Build history of the part. All positions in model axes, mm. Give positions to 0.01 mm unless a question says otherwise; leave off trailing zeros. Write each loop counter-clockwise with the first axis right and the second up, starting at its lowest first coordinate (ties: lowest second). Pieces come first, ordered by that corner, then holes.
from build123d import *

# Parameters (mm, degrees)
BOSS_EXTRUDE1_DEPTH = 25.4
CUT_EXTRUDE2_DEPTH  = 23.957211
SKETCH4_R           = 2.159
BOSS_EXTRUDE2_DEPTH = 7.62


with BuildPart() as part:
    # Sketch1 → Boss-Extrude1 (new body)
    with BuildSketch(Plane.XY):
        with BuildLine():
            ThreePointArc((-160.997616832, 14.9225), (-115.11071, 26.01979846), (-79.36572698, 56.858969015))
            ThreePointArc((-79.36572698, 56.858969015), (-44.613051666, 86.842020921), (0, 97.63125))
            Line((0, 97.63125), (0, 84.93125))
            ThreePointArc((0, 84.93125), (-58.347374184, 61.716295679), (-84.797616832, 4.7625))
            Line((-84.797616832, 4.7625), (-160.997616832, 4.7625))
            Line((-160.997616832, 4.7625), (-160.997616832, 14.9225))
        make_face()
    boss_extrude1 = extrude(amount=-BOSS_EXTRUDE1_DEPTH)

    # Sketch3 → Cut-Extrude2 (cut)
    with BuildSketch(Plane.XZ.offset(-4.7625)):
        with BuildLine():
            Line((-119.537512667, -16.51), (-110.197616832, -16.51))
            Line((-110.197616832, -16.51), (-110.197616832, -8.89))
            Line((-110.197616832, -8.89), (-119.537512667, -8.89))
            ThreePointArc((-119.537512667, -8.89), (-122.897616832, -7.62), (-126.257720997, -8.89))
            Line((-126.257720997, -8.89), (-135.597616832, -8.89))
            Line((-135.597616832, -8.89), (-135.597616832, -16.51))
            Line((-135.597616832, -16.51), (-126.257720997, -16.51))
            ThreePointArc((-126.257720997, -16.51), (-122.897616832, -17.78), (-119.537512667, -16.51))
        make_face()
    cut_extrude2 = extrude(amount=-CUT_EXTRUDE2_DEPTH, mode=Mode.SUBTRACT)

    # Mirror2: Boss-Extrude1, Cut-Extrude2 across plane
    add(boss_extrude1.mirror(Plane(origin=(0, 0, -25.4), x_dir=(0, 0, 1), z_dir=(-1, 0, 0))))
    add(cut_extrude2.mirror(Plane(origin=(0, 0, -25.4), x_dir=(0, 0, 1), z_dir=(-1, 0, 0))), mode=Mode.SUBTRACT)

    # Sketch4 → Boss-Extrude2 (add)
    with BuildSketch(Plane.XZ.offset(-4.7625)):
        with BuildLine():
            Line((-110.197616832, -8.89), (-119.537512667, -8.89))
            ThreePointArc((-119.537512667, -8.89), (-122.897616832, -7.62), (-126.257720997, -8.89))
            Line((-126.257720997, -8.89), (-135.597616832, -8.89))
            Line((-135.597616832, -8.89), (-135.597616832, -16.51))
            Line((-135.597616832, -16.51), (-126.257720997, -16.51))
            ThreePointArc((-126.257720997, -16.51), (-122.897616832, -17.78), (-119.537512667, -16.51))
            Line((-119.537512667, -16.51), (-110.197616832, -16.51))
            Line((-110.197616832, -16.51), (-110.197616832, -8.89))
        make_face()
        with Locations((-122.897616832, -12.7)):
            Circle(SKETCH4_R, mode=Mode.SUBTRACT)
    boss_extrude2 = extrude(amount=-BOSS_EXTRUDE2_DEPTH)

    # Mirror3: Boss-Extrude2 across plane
    add(boss_extrude2.mirror(Plane(origin=(0, 0, 0), x_dir=(0, 0, 1), z_dir=(1, 0, 0))))


solid = part.part
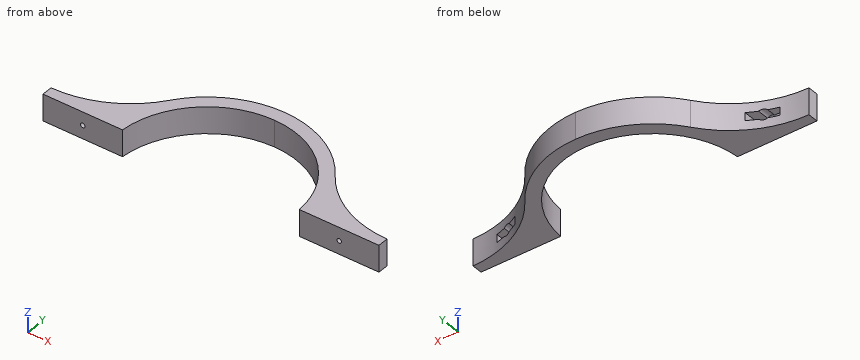
(1) Saw through at A-A, the plane y = 68.5. List the corners of the cut face in (x, z), plus the area to 3 significant figures.
(2) Saw through at B-B, the plane z = -3.75. List the corners of the cut face in (x, y).
(3) Drop flat-ended pins along their axis: pin 1 (3.5 mm diameter, centred on x = 122.9, z = -12.7, fed in from -Y); pin 2 (6 mm diameter, centred on y = 47.5, z = -15.5, fed in from -X); pin 3 (3 mm diameter, centred on y = 61.5, z = -22.5, fed in from +X); pin 4 (4 mm diameter, centred on y = 64.5, z = -8.5, fed in from -X). Give the stop position or say it passes through.
(4) Probe line 1 (Y direction, x = 112, z = -13); line 2 (X direction, y = 51, z = -12.75); line 3 (X direction, y = 61, z = -9.5). List the from-to ranges inside material, lowest first.
(5) Saw through at C-C, the plane y = 89. List the corners of the cut face in (x, z).
Computed values:
1. outline: (-69.57, -25.4) - (-50.21, -25.4) - (-50.21, 0) - (-69.57, 0) - close; (50.21, -25.4) - (69.57, -25.4) - (69.57, 0) - (50.21, 0) - close
1. area: 983 mm2
2. outline: (-161, 4.76) - (-84.8, 4.76) arc R84.93 cw to (84.8, 4.76) - (161, 4.76) - (161, 14.92) arc R100.42 cw to (79.37, 56.86) arc R97.63 ccw to (-79.37, 56.86) arc R100.42 cw to (-161, 14.92) - close
3. pin 1: passes through
3. pin 2: stops at x = -89.83
3. pin 3: stops at x = 77.02
3. pin 4: stops at x = -75
4. line 1: y = 4.76 to 12.38
4. line 2: x = -83.9 to -67.91, 67.91 to 83.9
4. line 3: x = -76.23 to -59.1, 59.1 to 76.23
5. outline: (-40.14, -25.4) - (40.14, -25.4) - (40.14, 0) - (-40.14, 0) - close
